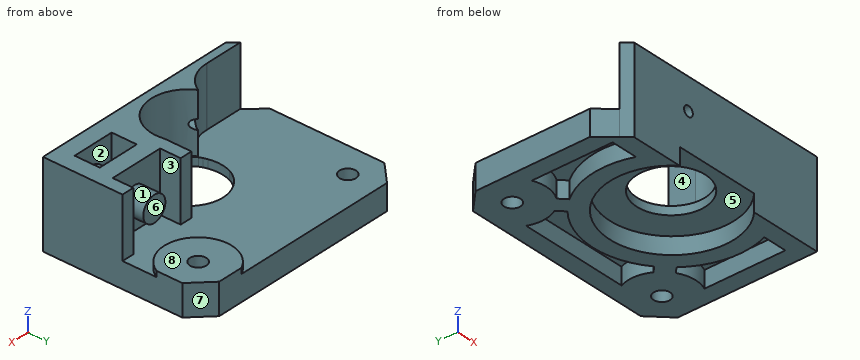
```python
from build123d import *

# Parameters (mm, degrees)
F0_W           = 7.551756
F0_H           = 4.45
F1_DEPTH       = 15.1
F0_R           = 1.45
F0_R_2         = 1.44
F2_DEPTH       = 4.5
F3_DEPTH       = 5.5
F4_R           = 11
F5_DEPTH       = 3
F6_R           = 2.25
F7_DEPTH       = 14
F8_D           = 1.79
F8_CBORE_D     = 1.79
F8_CBORE_DEPTH = 1.45


with BuildPart() as f1:
    # F0 (on Top) → F1 (new body)
    with BuildSketch(Plane.XY):
        with BuildLine():
            Line((2.65426, 1.450184), (3.954988, 0))
            Line((3.954988, 0), (41.2, 0))
            Line((41.2, 0), (41.2, 10.45))
            Line((41.2, 10.45), (41.2, 14.1))
            Line((41.2, 14.1), (39, 14.1))
            Line((39, 14.1), (39, 10.45))
            Line((39, 10.45), (29.35, 10.45))
            Line((29.35, 10.45), (29.35, 14.1))
            Line((29.35, 14.1), (27.15, 14.1))
            Line((27.15, 14.1), (27.15, 10.45))
            Line((27.15, 10.45), (27.15, 9.360534))
            ThreePointArc((27.15, 9.360534), (23.102126, 1.90917), (15.151799, 4.858818))
            ThreePointArc((15.151799, 4.858818), (12.818666, 2.347317), (9.508541, 1.45613))
            Line((9.508541, 1.45613), (9.425105, 1.450184))
            Line((9.425105, 1.450184), (2.65426, 1.450184))
        make_face()
        with Locations((34.424122, 5.225)):
            Rectangle(F0_W, F0_H, mode=Mode.SUBTRACT)
    extrude(amount=F1_DEPTH)

    # F0 (on Top) → F2 (join)
    with BuildSketch(Plane.XY):
        with BuildLine():
            Line((0, 4.409424), (2.65426, 1.450184))
            Line((2.65426, 1.450184), (9.425105, 1.450184))
            Line((9.425105, 1.450184), (9.508541, 1.45613))
            ThreePointArc((9.508541, 1.45613), (12.818666, 2.347317), (15.151799, 4.858818))
            ThreePointArc((15.151799, 4.858818), (23.102126, 1.90917), (27.15, 9.360534))
            Line((27.15, 9.360534), (27.15, 10.45))
            Line((27.15, 10.45), (27.15, 14.1))
            Line((27.15, 14.1), (29.35, 14.1))
            Line((29.35, 14.1), (29.35, 10.45))
            Line((29.35, 10.45), (39, 10.45))
            Line((39, 10.45), (39, 14.1))
            Line((39, 14.1), (41.2, 14.1))
            Line((41.2, 14.1), (41.2, 20.133845))
            ThreePointArc((41.2, 20.133845), (31.607359, 18.607359), (33.133845, 28.2))
            Line((33.133845, 28.2), (8.066155, 28.2))
            ThreePointArc((8.066155, 28.2), (9.592641, 18.607359), (0, 20.133845))
            Line((0, 20.133845), (0, 4.409424))
        make_face()
        with BuildLine():
            ThreePointArc((15.044259, 5.607124), (11.225264, 2.020343), (6.018226, 2.600408))
            ThreePointArc((6.018226, 2.600408), (4.726842, 11.501576), (13.680284, 12.358524))
            ThreePointArc((13.680284, 12.358524), (14.464459, 11.395564), (15.042763, 10.296571))
            ThreePointArc((15.042763, 10.296571), (15.139305, 10.532994), (15.245029, 10.765456))
            ThreePointArc((15.245029, 10.765456), (26.649775, 8.002179), (15.294389, 5.042598))
            ThreePointArc((15.294389, 5.042598), (15.162653, 5.321905), (15.044259, 5.607124))
        make_face(mode=Mode.SUBTRACT)
        with BuildLine():
            Line((0, 24.7), (0, 20.133845))
            ThreePointArc((0, 20.133845), (9.592641, 18.607359), (8.066155, 28.2))
            Line((8.066155, 28.2), (3.5, 28.2))
            Line((3.5, 28.2), (0, 24.7))
        make_face()
        with Locations((5.35, 22.85)):
            Circle(F0_R, mode=Mode.SUBTRACT)
        with BuildLine():
            ThreePointArc((13.680284, 12.358524), (4.726842, 11.501576), (6.018226, 2.600408))
            ThreePointArc((6.018226, 2.600408), (11.225264, 2.020343), (15.044259, 5.607124))
            ThreePointArc((15.044259, 5.607124), (14.926049, 5.938205), (14.825812, 6.275163))
            Line((14.825812, 6.275163), (14.824682, 6.275163))
            ThreePointArc((14.824682, 6.275163), (14.615506, 8.303124), (15.042763, 10.296571))
            ThreePointArc((15.042763, 10.296571), (14.464459, 11.395564), (13.680284, 12.358524))
        make_face()
        with Locations((9.25, 7.95)):
            Circle(F0_R_2, mode=Mode.SUBTRACT)
        with Locations((9.25, 7.95)):
            Circle(F0_R_2)
        with Locations((34.424122, 5.225)):
            Rectangle(F0_W, F0_H)
    extrude(amount=F2_DEPTH)

    # F0 (on Top) → F3 (join)
    with BuildSketch(Plane.XY):
        with BuildLine():
            ThreePointArc((33.133845, 28.2), (31.607359, 18.607359), (41.2, 20.133845))
            Line((41.2, 20.133845), (41.2, 24.7))
            Line((41.2, 24.7), (37.7, 28.2))
            Line((37.7, 28.2), (33.133845, 28.2))
        make_face()
        with Locations((35.85, 22.85)):
            Circle(F0_R, mode=Mode.SUBTRACT)
    extrude(amount=F3_DEPTH)

    # F4 (on Top) → F5 (cut)
    with BuildSketch(Plane.XY):
        with BuildLine():
            ThreePointArc((8.513082, 17.748509), (5.805837, 16.873794), (3, 17.344523))
            Line((3, 17.344523), (3, 3))
            Line((3, 3), (7.743291, 3))
            ThreePointArc((7.743291, 3), (6.98063, 10.038164), (9.758824, 16.549619))
            Line((9.758824, 16.549619), (8.513082, 17.748509))
        make_face()
        with Locations((20.828264, 7.978301)):
            Circle(F4_R)
        with BuildLine():
            Line((38.2, 3), (38.2, 17.33704))
            ThreePointArc((38.2, 17.33704), (35.445261, 16.871427), (32.77831, 17.703745))
            Line((32.77831, 17.703745), (31.773144, 16.708111))
            ThreePointArc((31.773144, 16.708111), (34.660709, 10.137804), (33.913237, 3))
            Line((33.913237, 3), (38.2, 3))
        make_face()
        with BuildLine():
            ThreePointArc((30.667119, 19.835147), (29.862233, 22.47726), (30.326221, 25.2))
            Line((30.326221, 25.2), (10.891282, 25.2))
            ThreePointArc((10.891282, 25.2), (11.357854, 22.520378), (10.593366, 19.910087))
            Line((10.593366, 19.910087), (11.839107, 18.711197))
            ThreePointArc((11.839107, 18.711197), (20.727473, 21.977938), (29.661953, 18.839513))
            Line((29.661953, 18.839513), (30.667119, 19.835147))
        make_face()
    extrude(amount=F5_DEPTH, mode=Mode.SUBTRACT)

    # F6 (on Front) → F7 (join)
    with BuildSketch(Plane.XZ):
        with Locations((34.6, 9.55)):
            Circle(F6_R)
    extrude(amount=-F7_DEPTH)

    # F8 (through all)
    with Locations(Plane.XZ):
        with Locations((15, 9.55)):
            CounterBoreHole(F8_D / 2, F8_CBORE_D / 2, F8_CBORE_DEPTH)


solid = f1.part
```
Check sheet for the modelled part. Datum: model origin and axes. Units: mm. Face numbers are marked on the shaded views. A direction names the side the tool comes from. Coordinates: 2 decimals unless noted, no trailing zeros. Loops run counter-clockwise (first coordinate to the right, second up) from the corner with the lowest first, then second, coordinate; pieces in that order, holes last. Notation, with made-up numbers: M 29.5,64 L 83.5,64 A30 ccw 83.5,97 Z; hole C 12,34 d2. An arc over 180 degrees is marked long. Answer as a JSON object with one key per item and string values.
1. Release check for a two-part mould opening along X. For the marked faces 5, 6, 7 and 8 record: pulls with the +X half, pulls with the -X half, needs draft (parallel to the pull), parting line crosses it, or undercut.
Outcome:
{"face 5": "undercut", "face 6": "undercut", "face 7": "pulls with the +X half", "face 8": "needs draft"}
2. Scan lines: L1, parallel to X at y = 12.25, z = 9.5; L2, parallel to Y at x = 35.85, z = 3.1; L3, parallel to Y at x = 35.85, z = 2.8. Record each from-to range of solid material in increasing order. Write a range as from..to.
Outcome:
{"L1": "27.15..29.35, 32.35..36.85, 39..41.2", "L2": "0..21.4, 24.3..28.2", "L3": "0..3, 16.86..21.4, 24.3..28.2"}
3. Sectioned sample at A-A on x = 35.85. Record the cut outline in (y, z), and give its area (3 significant figures).
Outcome:
{"outline": "M 0,0 L 3,0 L 3,3 L 16.86,3 L 16.86,0 L 21.4,0 L 21.4,5.5 L 16.85,5.5 L 16.85,4.5 L 10.45,4.5 L 10.45,7.68 L 14,7.68 L 14,11.42 L 10.45,11.42 L 10.45,15.1 L 7.45,15.1 L 7.45,11.42 L 3,11.42 L 3,15.1 L 0,15.1 Z; M 24.3,0 L 28.2,0 L 28.2,5.5 L 24.3,5.5 Z; hole M 3,4.5 L 7.45,4.5 L 7.45,7.68 L 3,7.68 Z", "area": "174 mm²"}
4. Access from +Z, -Z, +X, -X, +Y, -Y to the whole of each face (thin tool, end or side, straight path). Record for the marked faces 1, 2, 3 and 4.
Outcome:
{"face 1": "+Y", "face 2": "none", "face 3": "+Z, +Y", "face 4": "+Z, -X, +Y"}
5. Sectioned sample at B-B on y = 22.85. Record the cut outline in (x, z).
Outcome:
{"outline": "M 0,0 L 3.9,0 L 3.9,4.5 L 0,4.5 Z; M 6.8,0 L 11.37,0 L 11.37,3 L 29.85,3 L 29.85,0 L 34.4,0 L 34.4,5.5 L 29.85,5.5 L 29.85,4.5 L 6.8,4.5 Z; M 37.3,0 L 41.2,0 L 41.2,5.5 L 37.3,5.5 Z"}
6. Sectioned sample at D-D on x = 18. Record the cut outline in (y, z), and give its area (3 significant figures).
Outcome:
{"outline": "M 0,3 L 2.49,3 L 2.49,4.5 L 2.15,4.5 L 2.15,15.1 L 0,15.1 Z; M 13.41,3 L 18.61,3 L 18.61,0 L 21.69,0 L 21.69,3 L 25.2,3 L 25.2,0 L 28.2,0 L 28.2,4.5 L 13.41,4.5 Z", "area": "66.9 mm²"}
7. Sectioned sample at C-C on z = 9.55. Record the cut outline in (x, y) (3 decimals).
Outcome:
{"outline": "M 2.654,1.45 L 3.955,0 L 14.105,0 L 14.105,3.378 A6.211 cw 9.509,1.456 L 9.425,1.45 Z; M 15.895,0 L 41.2,0 L 41.2,14.1 L 39,14.1 L 39,10.45 L 36.85,10.45 L 36.85,14 L 32.35,14 L 32.35,10.45 L 29.35,10.45 L 29.35,14.1 L 27.15,14.1 L 27.15,9.361 A6.473 cw 15.895,3.779 Z; hole M 30.648,3 L 32.35,3 L 32.35,7.45 L 30.648,7.45 Z; hole M 36.85,3 L 38.2,3 L 38.2,7.45 L 36.85,7.45 Z"}
8. Depth check by flat-ended pin: P1, Ø1, axis at x = 36, y = 25, coming from the +Z side; P2, Ø3.5, axis at x = 35, z = 10, coming from the +Y side; P3, Ø1.4, axis at y = 12, z = 9, coming from the -X side. Enter the tip coordinate at first touch or a pass-through.
Outcome:
{"P1": "z = 5.5", "P2": "y = 14", "P3": "x = 27.15"}
